from build123d import *

# Parameters (mm, degrees)
BOSS_EXTRUDE1_DEPTH          = 38
FILLET3_R                    = 2
CUT_EXTRUDE1_DEPTH           = 98.450613347
CUT_EXTRUDE1_DEPTH_BACK      = 98.450613347
M3X0_5_TAPPED_HOLE3_D        = 2.5
M3X0_5_TAPPED_HOLE3_DEPTH    = 7.5
M3X0_5_TAPPED_HOLE3_TIP      = 0.751075774
M3X0_5_TAPPED_HOLE4_D        = 2.5
M3X0_5_TAPPED_HOLE4_DEPTH    = 7.5
M3X0_5_TAPPED_HOLE4_TIP      = 0.751075774
M2_5X0_45_TAPPED_HOLE1_D     = 2.05
M2_5X0_45_TAPPED_HOLE1_DEPTH = 6.35
M2_5X0_45_TAPPED_HOLE1_TIP   = 0.615882135
M2_5X0_45_TAPPED_HOLE2_D     = 2.05
M2_5X0_45_TAPPED_HOLE2_DEPTH = 6.35
M2_5X0_45_TAPPED_HOLE2_TIP   = 0.615882135
SKETCH14_R                   = 5
CUT_EXTRUDE2_DEPTH           = 98.58904673
SKETCH16_W                   = 6
SKETCH16_H                   = 6
BOSS_EXTRUDE2_DEPTH          = 4
FILLET4_R                    = 2
M3X0_5_TAPPED_HOLE5_D        = 2.5
M3X0_5_TAPPED_HOLE5_DEPTH    = 5.5
M3X0_5_TAPPED_HOLE5_TIP      = 0.751075774


with BuildPart() as part:
    # Sketch2 → Boss-Extrude1 (new body)
    with BuildSketch(Plane.XY.offset(11.2)):
        Polygon((-84.06534388, 85.95185693), (-75.56534388, 85.95185693), (-75.56534388, 82.95185693), (-5.56534388, 82.95185693), (-5.56534388, 85.95185693), (2.93465612, 85.95185693), (2.93465612, 79.95185693), (-84.06534388, 79.95185693), align=None)
    extrude(amount=BOSS_EXTRUDE1_DEPTH)

    # Fillet3
    fillet3_edges = [part.edges().sort_by_distance(p)[0] for p in [
        (2.93465612, 82.95185693, 49.2),
        (-84.06534388, 82.95185693, 11.2),
        (-84.06534388, 82.95185693, 49.2),
        (2.93465612, 82.95185693, 11.2),
    ]]
    fillet(fillet3_edges, radius=FILLET3_R)

    # Sketch3 → Cut-Extrude1 (cut, two sides: drawn at the far end of the back side and taken through both)
    with BuildSketch(Plane(origin=(0, 82.95185693, 0), x_dir=(1, 0, 0), z_dir=(0, 1, 0)).offset(-CUT_EXTRUDE1_DEPTH_BACK)):
        with BuildLine():
            Line((-66.06534388, -42.7), (-30.06534388, -42.7))
            ThreePointArc((-30.06534388, -42.7), (-17.56534388, -30.2), (-30.06534388, -17.7))
            Line((-30.06534388, -17.7), (-66.06534388, -17.7))
            ThreePointArc((-66.06534388, -17.7), (-78.56534388, -30.2), (-66.06534388, -42.7))
        make_face()
    extrude(amount=CUT_EXTRUDE1_DEPTH + CUT_EXTRUDE1_DEPTH_BACK, mode=Mode.SUBTRACT)

    # M3x0.5 Tapped Hole3
    with Locations(Plane.XY.offset(49.2)):
        with Locations((-78.56534388, 82.95185693), (-2.56534388, 82.95185693)):
            Hole(M3X0_5_TAPPED_HOLE3_D / 2, depth=M3X0_5_TAPPED_HOLE3_DEPTH)
            with Locations((0, 0, -(M3X0_5_TAPPED_HOLE3_DEPTH + M3X0_5_TAPPED_HOLE3_TIP / 2))):  # 118° drill point
                Cone(0, M3X0_5_TAPPED_HOLE3_D / 2, M3X0_5_TAPPED_HOLE3_TIP, mode=Mode.SUBTRACT)

    # M3x0.5 Tapped Hole4
    with Locations(Plane(origin=(0, 0, 11.2), x_dir=(-1, 0, 0), z_dir=(0, 0, -1))):
        with Locations((2.56534388, 82.95185693), (78.56534388, 82.95185693)):
            Hole(M3X0_5_TAPPED_HOLE4_D / 2, depth=M3X0_5_TAPPED_HOLE4_DEPTH)
            with Locations((0, 0, -(M3X0_5_TAPPED_HOLE4_DEPTH + M3X0_5_TAPPED_HOLE4_TIP / 2))):  # 118° drill point
                Cone(0, M3X0_5_TAPPED_HOLE4_D / 2, M3X0_5_TAPPED_HOLE4_TIP, mode=Mode.SUBTRACT)

    # M2.5x0.45 Tapped Hole1
    with Locations(Plane.ZY.offset(84.06534388)):
        with Locations((23.2, 82.95185693), (37.2, 82.95185693)):
            Hole(M2_5X0_45_TAPPED_HOLE1_D / 2, depth=M2_5X0_45_TAPPED_HOLE1_DEPTH)
            with Locations((0, 0, -(M2_5X0_45_TAPPED_HOLE1_DEPTH + M2_5X0_45_TAPPED_HOLE1_TIP / 2))):  # 118° drill point
                Cone(0, M2_5X0_45_TAPPED_HOLE1_D / 2, M2_5X0_45_TAPPED_HOLE1_TIP, mode=Mode.SUBTRACT)

    # M2.5x0.45 Tapped Hole2
    with Locations(Plane(origin=(2.93465612, 0, 0), x_dir=(0, 0, -1), z_dir=(1, 0, 0))):
        with Locations((-37.2, 82.95185693), (-23.2, 82.95185693)):
            Hole(M2_5X0_45_TAPPED_HOLE2_D / 2, depth=M2_5X0_45_TAPPED_HOLE2_DEPTH)
            with Locations((0, 0, -(M2_5X0_45_TAPPED_HOLE2_DEPTH + M2_5X0_45_TAPPED_HOLE2_TIP / 2))):  # 118° drill point
                Cone(0, M2_5X0_45_TAPPED_HOLE2_D / 2, M2_5X0_45_TAPPED_HOLE2_TIP, mode=Mode.SUBTRACT)

    # Sketch14 → Cut-Extrude2 (cut, through all)
    with BuildSketch(Plane(origin=(0, 85.95185693, 0), x_dir=(1, 0, 0), z_dir=(0, 1, 0))):
        with Locations(Location((-5.56534388, -30.2, 0), (0, 0, 270))):
            Circle(SKETCH14_R)
    extrude(amount=-CUT_EXTRUDE2_DEPTH, mode=Mode.SUBTRACT)

    # Sketch16 → Boss-Extrude2 (add)
    with BuildSketch(Plane.XZ.offset(-79.95185693)):
        with Locations((-81.06534388, 46.2)):
            Rectangle(SKETCH16_W, SKETCH16_H)
        with Locations((-81.06534388, 14.2)):
            Rectangle(SKETCH16_W, SKETCH16_H)
        with Locations((-15.06534388, 46.2)):
            Rectangle(SKETCH16_W, SKETCH16_H)
        with Locations((-15.06534388, 14.2)):
            Rectangle(SKETCH16_W, SKETCH16_H)
    extrude(amount=BOSS_EXTRUDE2_DEPTH)

    # Fillet4
    fillet4_edges = [part.edges().sort_by_distance(p)[0] for p in [
        (-12.06534388, 77.95185693, 49.2),
        (-12.06534388, 77.95185693, 11.2),
        (-84.06534388, 77.95185693, 11.2),
        (-84.06534388, 77.95185693, 49.2),
        (-78.06534388, 77.95185693, 43.2),
        (-78.06534388, 77.95185693, 17.2),
        (-18.06534388, 77.95185693, 17.2),
        (-18.06534388, 77.95185693, 43.2),
    ]]
    fillet(fillet4_edges, radius=FILLET4_R)

    # M3x0.5 Tapped Hole5
    with Locations(Plane.XZ.offset(-75.95185693)):
        with Locations((-81.06534388, 46.2), (-81.06534388, 14.2), (-15.06534388, 14.2), (-15.06534388, 46.2)):
            Hole(M3X0_5_TAPPED_HOLE5_D / 2, depth=M3X0_5_TAPPED_HOLE5_DEPTH)
            with Locations((0, 0, -(M3X0_5_TAPPED_HOLE5_DEPTH + M3X0_5_TAPPED_HOLE5_TIP / 2))):  # 118° drill point
                Cone(0, M3X0_5_TAPPED_HOLE5_D / 2, M3X0_5_TAPPED_HOLE5_TIP, mode=Mode.SUBTRACT)


solid = part.part
Geometry check sheet. Reference: the model listing, model coordinates, mm. A direction names the side the tool comes from. Round coordinates to 2 decimals unless told otherwise and drop trailing zeros. Loops run counter-clockwise (first coordinate to the right, second up) from the corner with the lowest first, then second, coordinate; pieces in that order, holes last.
Item 1: Cross-section at A-A on y = 78.25. Record the boundary of the cut face in (x, z), then the cut area to 3 significant figures.
Item 2: Cross-section at C-C on z = 39.5. Record the boundary of the cut face in (x, y), then the cut area to 3 significant figures.
Item 3: Cross-section at D-D on x = -71. Record the boundary of the cut face in (y, z).
Item 4: Access from +Z, -Z, +X, -X, +Y, -Y to the whole of each face (thin tool, end or side, straight path). Record for faces 4 (the flat face through (-78.065, 78, 13)), 5 (the cylindrical face through (-2.4, 84.19, 45.4)), 6 (the flat face through (-30, 79.952, 17)).
Item 5: Thickness scan on line 1 (X direction, y = 85.75, z = 44.5); line 2 (Z direction, x = -45, y = 82); line 3 (Y direction, x = -80.75, z = 37.2). Record the ranges inside material, lowest first.
Item 6: Mould release check, pull along Z, two halves, no side actions. Record for faces 1 (the conical face through (-3.924, 82.96, 23.378)), 2 (the flat face through (-78.065, 78, 47)), 3 (the cylindrical face through (2.364, 82.91, 48.599)): pulls with the +Z half, pulls with the -Z half, needs draft (parallel to the pull), parting line crosses it, or undercut.
Item 7: Gauge pin test, flat ends, axial feed: pin 1 (4.5 mm diameter, centred on x = -82.5, y = 77.5, fed in from -Z); pin 2 (5 mm diameter, centred on x = -45.5, z = 42.5, fed in from -Y); pin 3 (12 mm diameter, centred on x = -39.5, z = 34, fed in from +Y); pin 4 (1.6 mm diameter, centred on y = 82.95, z = 23.2, fed in from +X). Record the tip position at first contact, or that the pin passes through.
Item 8: Cross-section at B-B on x = -34. Record the boundary of the cut face in (y, z), then the cut area to 3 significant figures.
Answer sheet:
1. outline: (-84.07, 13.2) arc R2 ccw to (-82.07, 11.2) - (-78.07, 11.2) - (-78.07, 15.2) arc R2 ccw to (-80.07, 17.2) - (-84.07, 17.2) - close; (-84.07, 43.2) - (-80.07, 43.2) arc R2 ccw to (-78.07, 45.2) - (-78.07, 49.2) - (-82.07, 49.2) arc R2 ccw to (-84.07, 47.2) - close; (-18.07, 11.2) - (-14.07, 11.2) arc R2 ccw to (-12.07, 13.2) - (-12.07, 17.2) - (-16.07, 17.2) arc R2 ccw to (-18.07, 15.2) - close; (-18.07, 45.2) arc R2 ccw to (-16.07, 43.2) - (-12.07, 43.2) - (-12.07, 47.2) arc R2 ccw to (-14.07, 49.2) - (-18.07, 49.2) - close; hole circle Ø2.5 at (-81.07, 14.2); hole circle Ø2.5 at (-81.07, 46.2); hole circle Ø2.5 at (-15.07, 14.2); hole circle Ø2.5 at (-15.07, 46.2)
1. area: 117 mm2
2. outline: (-84.07, 79.95) - (-74.42, 79.95) - (-74.42, 82.95) - (-75.57, 82.95) - (-75.57, 85.95) - (-84.07, 85.95) - close; (-21.71, 79.95) - (2.93, 79.95) - (2.93, 85.95) - (-5.57, 85.95) - (-5.57, 82.95) - (-21.71, 82.95) - close
2. area: 154 mm2
3. outline: (79.95, 11.2) - (82.95, 11.2) - (82.95, 18.72) - (79.95, 18.72) - close; (79.95, 41.68) - (82.95, 41.68) - (82.95, 49.2) - (79.95, 49.2) - close
4. face 4: +Z, -Z, -Y
4. face 5: +Z
4. face 6: -Y
5. line 1: x = -84.07 to -75.57, -5.57 to 2.93
5. line 2: z = 11.2 to 17.7, 42.7 to 49.2
5. line 3: y = 79.95 to 81.93, 83.98 to 85.95
6. face 1: undercut
6. face 2: needs draft
6. face 3: pulls with the +Z half
7. pin 1: stops at z = 11.2
7. pin 2: stops at y = 79.95
7. pin 3: passes through
7. pin 4: stops at x = -3.55
8. outline: (79.95, 11.2) - (82.95, 11.2) - (82.95, 17.7) - (79.95, 17.7) - close; (79.95, 42.7) - (82.95, 42.7) - (82.95, 49.2) - (79.95, 49.2) - close
8. area: 39.0 mm2
